Design review of the part built by this model. Coordinates are the model's own, in mm. A direction names the side the tool comes from. Give positions to 0.01 mm unless a question says otherwise; leave off trailing zeros. Loops run counter-clockwise (first coordinate to the right, second up) from the corner with the lowest first, then second, coordinate; pieces in that order, holes last. Notation, with made-up numbers: (30.25, -35) -> (88.25, -35) arc R9 cw to (88.25, -21) -> close; hole circle Ø3 at (85, 6.5). An arc over 180 degrees is marked (long way). Answer in a Markdown table with one row per item. Add a question column.
(1) For line 1 (X direction, y = 6, z = 2.5); line 2 (X direction, y = 2.5, z = 8.75); line 3 (Y direction, x = -17.5, z = 3.5), list the stretches that pass through material, from the lowest coordinate up.
(2) For pin 1 (4 mm diameter, centred on x = -15, z = 4.5, fed in from +Y); pin 2 (10 mm diameter, centred on x = 8.5, z = 13.5, fed in from -Y); pin 3 (1 mm diameter, centred on y = 1.5, z = 15, fed in from -X), all flat-tipped, find the tip position at first contact; note any pin that passes through.
(3) For faces 1 (the flat face through (26, 1, 17)), 2 (the flat face through (32, 6, 2)), 3 (the flat face through (-25.49, 0.51, 16.02)), 4 (the flat face through (27.5, 1, 16)), list the 3-axis set-ups (+Z, -Z, +X, -X, +Y, -Y) from which the entire face can be reached by the end or side of a thin tool; tool diameter is ignored.
(4) Consider section A-A on z = 16. Write out the cut boundary in (x, y).
(5) Consider section B-B on y = 6.5. Write out the cut boundary in (x, z), then the cut area to 3 significant figures.
(6) Draft analysis for pull direction X (two halves, no side actions). For faces 5 (the flat face through (26.99, 1.02, 13.99)), 6 (the flat face through (6, 2, 3.3)), 7 (the flat face through (-27.5, 2, 16)), state which applies: +X half, -X half, draft (parallel to the pull), parting line (faces both ways), or undercut.
(7) Consider section D-D on z = 1.5. Write out the cut boundary in (x, y).
(8) Consider section C-C on x = -8. Write out the cut boundary in (y, z), then the cut area to 3 significant figures.
from build123d import *

# Parameters (mm, degrees)
PAD_DEPTH       = 4
SKETCH001_W     = 53
SKETCH001_H     = 1
POCKET_DEPTH    = 1
SKETCH002_W     = 3
SKETCH002_H     = 1
PAD001_DEPTH    = 13
PAD002_DEPTH    = 2
SKETCH004_W     = 1
SKETCH004_H     = 3
PAD003_DEPTH    = 2
CHAMFER_SIZE    = 1.99
SKETCH005_W     = 1
SKETCH005_H     = 1
PAD004_DEPTH    = 2
CHAMFER001_SIZE = 1.99
CHAMFER002_SIZE = 0.99


with BuildPart() as part:
    # Sketch → Pad (new body)
    with BuildSketch(Plane.XY):
        Polygon((34.5, 10), (34.5, 0), (-34.5, 0), (-34.5, 10), (-32, 10), (-32, 3), (32, 3), (32, 10), align=None)
    extrude(amount=PAD_DEPTH)

    # Sketch001 (on Face10 of Pad) → Pocket (cut)
    with BuildSketch(Plane.XY.offset(4)):
        with Locations((0, 1.5)):
            Rectangle(SKETCH001_W, SKETCH001_H)
    extrude(amount=-POCKET_DEPTH, mode=Mode.SUBTRACT)

    # Sketch002 (on Face5 of Pocket) → Pad001 (join)
    with BuildSketch(Plane.XY.offset(4)):
        with Locations((-25, 2.5)):
            Rectangle(SKETCH002_W, SKETCH002_H)
        with Locations((25, 2.5)):
            Rectangle(SKETCH002_W, SKETCH002_H)
    extrude(amount=PAD001_DEPTH)

    # Sketch003 (on Face20 of Pad001) → Pad002 (join)
    with BuildSketch(Plane.XY.offset(17)):
        Polygon((-23.5, 3), (-27.5, 3), (-27.5, 0), (-24.5, 0), (-24.5, 1), (-26.5, 1), (-26.5, 2), (-23.5, 2), align=None)
        Polygon((27.5, 3), (23.5, 3), (23.5, 2), (26.5, 2), (26.5, 1), (24.5, 1), (24.5, 0), (27.5, 0), align=None)
    extrude(amount=PAD002_DEPTH)

    # Sketch004 (on Face20 of Pad002) → Pad003 (join)
    with BuildSketch(Plane(origin=(0, 0, 17), x_dir=(1, 0, 0), z_dir=(0, 0, -1))):
        with Locations((-27, -1.5)):
            Rectangle(SKETCH004_W, SKETCH004_H)
        with Locations((27, -1.5)):
            Rectangle(SKETCH004_W, SKETCH004_H)
    extrude(amount=PAD003_DEPTH)

    # Chamfer
    chamfer_edges = [part.edges().sort_by_distance(p)[0] for p in [
        (-26.5, 0.5, 17),
        (26.5, 0.5, 17),
    ]]
    chamfer(chamfer_edges, length=CHAMFER_SIZE)

    # Sketch005 (on Face4 of Chamfer) → Pad004 (join)
    with BuildSketch(Plane(origin=(0, 0, 15), x_dir=(1, 0, 0), z_dir=(0, 0, -1))):
        with Locations((-27, -2.5)):
            Rectangle(SKETCH005_W, SKETCH005_H)
        with Locations((27, -2.5)):
            Rectangle(SKETCH005_W, SKETCH005_H)
    extrude(amount=PAD004_DEPTH)

    # Chamfer001
    chamfer001_edges = [part.edges().sort_by_distance(p)[0] for p in [
        (27, 2, 15),
        (-27, 2, 15),
    ]]
    chamfer(chamfer001_edges, length=CHAMFER001_SIZE)

    # Chamfer002
    chamfer002_edges = [part.edges().sort_by_distance(p)[0] for p in [
        (-26.5, 2.5, 13),
        (26.5, 2.5, 13),
    ]]
    chamfer(chamfer002_edges, length=CHAMFER002_SIZE)


solid = part.part
Values follow:
| question | item | result |
|---|---|---|
| 1 | line 1 | -34.5 to -32, 32 to 34.5 |
| 1 | line 2 | -26.5 to -23.5, 23.5 to 26.5 |
| 1 | line 3 | 0 to 1, 2 to 3 |
| 2 | pin 1 | y = 3 |
| 2 | pin 2 | through |
| 2 | pin 3 | x = -27.5 |
| 3 | face 1 | +Z |
| 3 | face 2 | +Z, -Z, +Y |
| 3 | face 3 | -Y |
| 3 | face 4 | +Z, +X, +Y, -Y |
| 4 | outline | (-27.5, 0) -> (-25.51, 0) -> (-25.51, 1) -> (-26.5, 1) -> (-26.5, 2) -> (-23.5, 2) -> (-23.5, 3) -> (-27.5, 3) -> close; (23.5, 2) -> (26.5, 2) -> (26.5, 1) -> (25.51, 1) -> (25.51, 0) -> (27.5, 0) -> (27.5, 3) -> (23.5, 3) -> close |
| 5 | outline | (-34.5, 0) -> (-32, 0) -> (-32, 4) -> (-34.5, 4) -> close; (32, 0) -> (34.5, 0) -> (34.5, 4) -> (32, 4) -> close |
| 5 | area | 20.0 mm2 |
| 6 | face 5 | draft |
| 6 | face 6 | undercut |
| 6 | face 7 | -X half |
| 7 | outline | (-34.5, 0) -> (34.5, 0) -> (34.5, 10) -> (32, 10) -> (32, 3) -> (-32, 3) -> (-32, 10) -> (-34.5, 10) -> close |
| 8 | outline | (0, 0) -> (3, 0) -> (3, 4) -> (2, 4) -> (2, 3) -> (1, 3) -> (1, 4) -> (0, 4) -> close |
| 8 | area | 11.0 mm2 |
